Input: part model. Units: mm. Frame: model coordinates. A direction names the side the tool comes from. Give positions to 0.01 mm unless a question says otherwise; leave off trailing zeros. Write each loop counter-clockwise with the first axis right and the second up, starting at its lowest first coordinate (ties: lowest second). Pieces come first, ordered by that corner, then holes. Notation, with made-up numbers: (-2, 24) -> (6, 24) arc R9 cw to (6, 36) -> close; hole circle Ø9 at (80.25, 8). An arc over 180 degrees is marked (long way). Return JSON: item names as keys, results as strings. Group by question number.
Item 1: Pin query (flat end, axial travel): P1, Ø3, axis at x = -2, y = -10.5, coming from the -Z side; P2, Ø2, axis at y = 0, z = 1.5, coming from the -X side; P3, Ø0.7, axis at x = 0, y = 1, coming from the -Z side. Return the tip coordinate at first contact, or that it passes through.
Item 2: Mould query, pull axis Z, two halves, no side actions, for faces 1 (the face through (-1.5, -5.67, 0.07)), 2 (the face through (0.991, 1.26, 0.583)), 3 (the face through (0, -12, 0)). Classes: released by +Z, released by -Z, zero draft, split by the parting line, or undercut.
Item 3: Line query: line 1 (X direction, y = -9, z = 0.1); line 2 (X direction, y = 1, z = 2.15); line 3 (Y direction, x = 0.45, z = 0.8). Output: solid intervals per line, ascending. Write a range as [from, to].
Item 4: Set-up query: faces 4 (the face through (0, 1, 1.15)), 5 (the face through (0, 0, 2)). Return all of +Z, -Z, +X, -X, +Y, -Y with unobstructed straight access to the full face (end or side cutting, diameter ignored); none if empty.
Item 5: Section A-A, the plane y = -1.25. Return loops of the section in (x, z).
from build123d import *

# Parameters (mm, degrees)
FILLET_1_R          = 0.2
CUT_EXTRUDE_1_DEPTH = 1.5
SKETCH_3_R          = 1.5
EXTRUDE_1_DEPTH     = 12
CHAMFER_1_SIZE      = 0.5


with BuildPart() as part:
    # 草图1 → 旋转1 (revolve)
    with BuildSketch(Plane.XY):
        with BuildLine():
            Line((0, 0), (0, 2))
            Line((0, 2), (1.3, 2))
            ThreePointArc((1.3, 2), (2.370691821, 1.250626571), (2.75, 0))
            Line((2.75, 0), (0, 0))
        make_face()
    revolve(axis=Axis((0, 0, 0), (0, 1, 0)))

    # 圆角1
    fillet_1_edges = [part.edges().sort_by_distance(p)[0] for p in [
        (-2.75, 0, 0),
    ]]
    fillet(fillet_1_edges, radius=FILLET_1_R)

    # 草图2 → 切除-拉伸1 (cut)
    with BuildSketch(Plane(origin=(0, 2, 0), x_dir=(1, 0, 0), z_dir=(0, 1, 0))):
        Polygon((1.327905619, 0), (0.66395281, 1.15), (-0.66395281, 1.15), (-1.327905619, 0), (-0.66395281, -1.15), (0.66395281, -1.15), align=None)
    extrude(amount=-CUT_EXTRUDE_1_DEPTH, mode=Mode.SUBTRACT)

    # 草图3 → 凸台-拉伸1 (add)
    with BuildSketch(Plane.XZ):
        Circle(SKETCH_3_R)
    extrude(amount=EXTRUDE_1_DEPTH)

    # 倒角1
    chamfer_1_edges = [part.edges().sort_by_distance(p)[0] for p in [
        (-1.5, -12, 0),
    ]]
    chamfer(chamfer_1_edges, length=CHAMFER_1_SIZE)


solid = part.part
Answer below:
{
 "1": {"P1": "stops at z = -1.41", "P2": "stops at x = -2.7", "P3": "stops at z = -2.67"},
 "2": {"face 1": "split by the parting line", "face 2": "undercut", "face 3": "zero draft"},
 "3": {"line 1": "x = [-1.5, 1.5]", "line 2": "x = [-1.33, 1.33]", "line 3": "y = [-12, 0.5]"},
 "4": {"face 4": "+Y", "face 5": "-Y"},
 "5": {"outline": "circle Ø3 at (0, 0)"}
}
